Autodesk Inventor part; units mm, degrees
ref_plane "YZ Plane" through (0, 0, 0) normal (1, 0, 0) x (0, 1, 0)
ref_plane "XZ Plane" through (0, 0, 0) normal (0, 1, 0) x (-1, 0, 0)
ref_plane "XY Plane" through (0, 0, 0) normal (0, 0, 1) x (1, 0, 0)
sketch "Sketch1" plane through (0, 0, 0) normal (0, 1, 0) x (-1, 0, 0)
  line L0 (-25.2, 25.2) -> (25.2, 25.2)
  line L1 (25.2, 25.2) -> (25.2, -25.2)
  line L2 (25.2, -25.2) -> (-25.2, -25.2)
  line L3 (-25.2, -25.2) -> (-25.2, 25.2)
  line L4 (-25.2, 25.2) -> (25.2, -25.2) construction
  line L5 (25.2, 25.2) -> (-25.2, -25.2) construction
  line L6 (-50, 50) -> (50, 50)
  line L7 (50, 50) -> (50, -50)
  line L8 (50, -50) -> (-50, -50)
  line L9 (-50, -50) -> (-50, 50)
  line L10 (-50, 50) -> (50, -50) construction
  line L11 (50, 50) -> (-50, -50) construction
  point P0 (0, 0)
  dimension "d0" = 50.4
  dimension "d1" = 100
extrude "Extrusion1" add sketch "Sketch1" along normal blind 5
fillet "Fillet1" radius 5 8 edges at (50, 2.5, 50) (50, 2.5, -50) (-50, 2.5, 50) (-50, 2.5, -50) (-25.2, 2.5, -25.2) (25.2, 2.5, -25.2) (-25.2, 2.5, 25.2) (25.2, 2.5, 25.2)
properties part number "PATA" material "Steel, Mild, Welded"
Check sheet for the modelled part. Datum: model origin and axes. Units: mm. A direction names the side the tool comes from. Coordinates: 2 decimals unless noted, no trailing zeros. Write each loop counter-clockwise with the first axis right and the second up, starting at its lowest first coordinate (ties: lowest second). Pieces come first, ordered by that corner, then holes. Notation, with made-up numbers: M 27.25,-29.5 L 41.25,-29.5 A10 cw 41.25,-21.5 Z; hole C -25,86.5 d11. An arc over 180 degrees is marked long. Answer as CSV lines item,"result".
Q1. Material ranges on probe 1 along Z at (x, y) = (13.5, 0.8), recorded low to high. Write a range as from..to.
Check result:
probe 1,"-50..-25.2, 25.2..50"
Q2. Set-up check for faces 4 (the face through (0, 2, 25.2)), 5 (the face through (-50, 2, 1)): record each of +Z, -Z, +X, -X, +Y, -Y from which the full face is reachable in a straight line by a thin tool's end or side.
Check result:
face 4,"+Y, -Y"
face 5,"+Z, -Z, -X, +Y, -Y"
Q3. Cross-section at A-A (x = 14). Record the boundary of the cut face in (y, z).
Check result:
outline,"M 0,-50 L 5,-50 L 5,-25.2 L 0,-25.2 Z; M 0,25.2 L 5,25.2 L 5,50 L 0,50 Z"
Q4. Cross-section at B-B (y = 3.55). Record the boundary of the cut face in (x, z), then the cut area to 3 significant figures.
Check result:
outline,"M -50,-45 A5 ccw -45,-50 L 45,-50 A5 ccw 50,-45 L 50,45 A5 ccw 45,50 L -45,50 A5 ccw -50,45 Z; hole M -25.2,-20.2 A5 ccw -20.2,-25.2 L 20.2,-25.2 A5 ccw 25.2,-20.2 L 25.2,20.2 A5 ccw 20.2,25.2 L -20.2,25.2 A5 ccw -25.2,20.2 Z"
area,"7,460 mm^2"
Q5. Mould release check, pull along Z, two halves, no side actions. Record for faces 1 (the face through (-49, 3, 48)), 2 (the face through (-23.7, 2.54, -23.77)), 3 (the face through (-1, 2, -50)): released by +Z, released by -Z, zero draft, split by the parting line, or undercut.
Check result:
face 1,"released by +Z"
face 2,"undercut"
face 3,"released by -Z"
Q6. Cross-section at C-C (z = -4). Record the boundary of the cut face in (x, y).
Check result:
outline,"M -50,0 L -25.2,0 L -25.2,5 L -50,5 Z; M 25.2,0 L 50,0 L 50,5 L 25.2,5 Z"
